Check sheet for the modelled part. Datum: model origin and axes. Units: mm. A direction names the side the tool comes from. Give positions to 0.01 mm unless a question says otherwise; leave off trailing zeros. Write each loop counter-clockwise with the first axis right and the second up, starting at its lowest first coordinate (ties: lowest second). Pieces come first, ordered by that corner, then holes. Notation, with made-up numbers: (18.5, 59) -> (29.5, 59) arc R15 cw to (29.5, 72) -> close; hole circle Ø6 at (84, 31). An arc over 180 degrees is marked (long way). Use a Markdown table: item, result. Add a question column.
1. Cross-section at C-C (z = -31.5). Enter the section's corners in (x, y), then the cut area to 3 significant figures.
2. Cross-section at D-D (x = 5.5). Enter the section's corners in (y, z).
3. Release check for a two-part mould opening along Y. For faces 6 (the flat face through (3, 0, -24)), 7 (the cylindrical face through (4.077, 3.391, -24.692)), 8 (the flat face through (2, 14, -12)) record: released by +Y, released by -Y, zero draft, split by the parting line, or undercut.
4. Cross-section at B-B (y = 4.5). Enter the section's corners in (x, z), then the cut area to 3 significant figures.
5. Scan lines: probe 1 along Y at (x, z) = (3.5, -26.5); probe 2 along Y at (x, z) = (3.5, -2.1); probe 3 along X at (y, z) = (4.75, -14). Record each from-to range of solid material in increasing order. Write a range as [from, to].
6. Cross-section at A-A (x = 3.5). Enter the section's corners in (y, z).
7. Set-up check for faces 1 (the flat face through (0, 5, -23)), 2 (the flat face through (4, 6, -3)), 3 (the flat face through (2, 14, -5)), 4 (the flat face through (3, 3, -47)), 5 (the flat face through (4.5, 14, -8)): record each of +Z, -Z, +X, -X, +Y, -Y from which the full face is reachable in a straight line by a thin tool's end or side.
8. Gauge pin test, flat ends, axial feed: P1, Ø3.5, axis at y = 15.5, z = -7, coming from the +X side; P2, Ø1.3, axis at x = 2, y = 13.5, coming from the +Z side; P3, Ø2, axis at x = 3, y = 16, coming from the -Z side. Record the tip position at first contact, or that the pin passes through.
from build123d import *

# Parameters (mm, degrees)
CROQUIS1_W              = 7
CROQUIS1_H              = 47
SALIENTE_EXTRUIR1_DEPTH = 9
CROQUIS2_W              = 4.5
CROQUIS2_H              = 7
SALIENTE_EXTRUIR2_DEPTH = 10
CROQUIS3_R              = 1.25
CORTAR_EXTRUIR1_DEPTH   = 49
CROQUIS6_R              = 2.5
CORTAR_EXTRUIR2_DEPTH   = 3


with BuildPart() as part:
    # Croquis1 → Saliente-Extruir1 (new body)
    with BuildSketch(Plane(origin=(0, 0, 0), x_dir=(1, 0, 0), z_dir=(0, 1, 0))):
        with Locations((3.5, 23.5)):
            Rectangle(CROQUIS1_W, CROQUIS1_H)
    extrude(amount=SALIENTE_EXTRUIR1_DEPTH)

    # Croquis2 → Saliente-Extruir2 (add)
    with BuildSketch(Plane(origin=(0, 9, 0), x_dir=(1, 0, 0), z_dir=(0, 1, 0))):
        with Locations((2.25, 8.5)):
            Rectangle(CROQUIS2_W, CROQUIS2_H)
    extrude(amount=SALIENTE_EXTRUIR2_DEPTH)

    # Croquis3 → Cortar-Extruir1 (cut)
    with BuildSketch(Plane.XY):
        with Locations((3.5, 4.5)):
            Circle(CROQUIS3_R)
    extrude(amount=-CORTAR_EXTRUIR1_DEPTH, mode=Mode.SUBTRACT)

    # Croquis6 → Cortar-Extruir2 (cut)
    with BuildSketch(Plane.XY):
        with Locations((3.5, 4.5)):
            Circle(CROQUIS6_R)
    extrude(amount=-CORTAR_EXTRUIR2_DEPTH, mode=Mode.SUBTRACT)


solid = part.part
Worked answers:
| question | item | result |
|---|---|---|
| 1 | outline | (0, 0) -> (7, 0) -> (7, 9) -> (0, 9) -> close; hole circle Ø2.5 at (3.5, 4.5) |
| 1 | area | 58.1 mm² |
| 2 | outline | (0, -47) -> (9, -47) -> (9, 0) -> (6, 0) -> (6, -3) -> (3, -3) -> (3, 0) -> (0, 0) -> close |
| 3 | face 6 | released by -Y |
| 3 | face 7 | undercut |
| 3 | face 8 | zero draft |
| 4 | outline | (0, -47) -> (2.25, -47) -> (2.25, -3) -> (1, -3) -> (1, 0) -> (0, 0) -> close; (4.75, -47) -> (7, -47) -> (7, 0) -> (6, 0) -> (6, -3) -> (4.75, -3) -> close |
| 4 | area | 204 mm² |
| 5 | probe 1 | y = [0, 3.25], [5.75, 9] |
| 5 | probe 2 | y = [0, 2], [7, 9] |
| 5 | probe 3 | x = [0, 2.28], [4.72, 7] |
| 6 | outline | (0, -47) -> (3.25, -47) -> (3.25, -3) -> (2, -3) -> (2, 0) -> (0, 0) -> close; (5.75, -47) -> (9, -47) -> (9, -12) -> (19, -12) -> (19, -5) -> (9, -5) -> (9, 0) -> (7, 0) -> (7, -3) -> (5.75, -3) -> close |
| 7 | face 1 | +Z, -Z, -X, +Y, -Y |
| 7 | face 2 | +Z |
| 7 | face 3 | +Z, +X, -X, +Y |
| 7 | face 4 | -Z, +X, -X, +Y, -Y |
| 7 | face 5 | +Z, -Z, +X, +Y |
| 8 | P1 | stops at x = 4.5 |
| 8 | P2 | stops at z = -5 |
| 8 | P3 | stops at z = -12 |
